```python
from build123d import *

# Parameters (mm, degrees)
F0_W      = 63.5
F0_H      = 6.35
F1_DEPTH  = 38.1
F2_W      = 25.4
F2_H      = 38.1
F3_DEPTH  = 12.7
F5_DEPTH  = 25.4
F6_R      = 6.35
F7_DEPTH  = 25.4
F9_DEPTH  = 25.4
F11_DEPTH = 12.7
F12_R     = 3.4395833333
F13_DEPTH = 25.4
F14_DEPTH = 25.4


with BuildPart() as f1:
    # F0 (on Front) → F1 (new body)
    with BuildSketch(Plane.XZ):
        with Locations((-14.0939018427, 3.175)):
            Rectangle(F0_W, F0_H)
    extrude(amount=F1_DEPTH)

    # F2 (on face) → F3 (join)
    with BuildSketch(Plane(origin=(0, 0, 0), x_dir=(-1, 0, 0), z_dir=(0, 1, 0))):
        with Locations((33.1439018427, 25.4)):
            Rectangle(F2_W, F2_H)
    extrude(amount=-F3_DEPTH)

    # F4 (on face) → F5 (cut)
    with BuildSketch(Plane.XZ.offset(12.7)):
        with BuildLine():
            ThreePointArc((-45.8439018427, 25.4), (-33.1439018427, 38.1), (-20.4439018427, 25.4))
            Line((-20.4439018427, 25.4), (-20.4439018427, 44.45))
            Line((-20.4439018427, 44.45), (-45.8439018427, 44.45))
            Line((-45.8439018427, 44.45), (-45.8439018427, 25.4))
        make_face()
    extrude(amount=-F5_DEPTH, mode=Mode.SUBTRACT)

    # F6 (on face) → F7 (cut)
    with BuildSketch(Plane.XZ.offset(12.7)):
        with Locations((-33.1439018427, 25.4)):
            Circle(F6_R)
    extrude(amount=-F7_DEPTH, mode=Mode.SUBTRACT)

    # F8 (on face) → F9 (cut)
    with BuildSketch(Plane.XZ.offset(12.7)):
        with BuildLine():
            add(Edge.make_bspline(
                [(-20.4439018427, 25.4), (-21.2112794526, 20.9739528082), (-22.6711814471, 15.8700383759), (-20.4439018427, 12.7)],
                knots=[0, 0, 0, 0, 0.4860571438, 0.4860571438, 0.4860571438, 0.4860571438], degree=3))
            Line((-20.4439018427, 12.7), (-20.4439018427, 25.4))
        make_face()
    extrude(amount=-F9_DEPTH, mode=Mode.SUBTRACT)

    # F10 (on face) → F11 (join)
    with BuildSketch(Plane.XZ.offset(12.7)):
        with BuildLine():
            add(Edge.make_bspline(
                [(-20.4439018427, 12.7), (-18.2158628234, 9.3571333053), (-12.2381824129, 8.0261796099), (-7.7439018427, 6.35)],
                knots=[0.4860571438, 0.4860571438, 0.4860571438, 0.4860571438, 1, 1, 1, 1], degree=3))
            Line((-20.4439018427, 12.7), (-20.4439018427, 6.35))
            Line((-20.4439018427, 6.35), (-7.7439018427, 6.35))
        make_face()
    extrude(amount=-F11_DEPTH)

    # F12 (on face) → F13 (cut)
    with BuildSketch(Plane.XY.offset(6.35)):
        with Locations((8.1310981573, -9.2604166667)):
            Circle(F12_R)
    extrude(amount=-F13_DEPTH, mode=Mode.SUBTRACT)

    # F14 (cut): a face of the model
    f14_faces = [f1.faces().sort_by_distance(p)[0] for p in [
        (-11.2918846227, -22.4788355031, 6.35),
    ]]
    extrude(f14_faces, amount=-F14_DEPTH, mode=Mode.SUBTRACT)


solid = f1.part
```
Source: CAD feature listing. Evaluate the final solid. Frame: model axes, mm. Coordinates: 2 decimals unless noted, no trailing zeros. Loops run counter-clockwise (first coordinate to the right, second up) from the corner with the lowest first, then second, coordinate; pieces in that order, holes last. Notation, with made-up numbers: M 76,-22.5 L 91,-22.5 A17 ccw 91,-11.5 Z; hole C 32.25,88.25 d10. An arc over 180 degrees is marked long. Use CSV: the item, a comma, the result in double quotes.
(1) Draft query along Z for faces 1 (the face through (-31, -12.7, 15)), 2 (the face through (-38.183, -6.439, 21.536)), 3 (the face through (-27, -6, 0)). Return one class per face: pulls with the +Z half, pulls with the -Z half, needs draft (parallel to the pull), parting line crosses it, or undercut.
Answers follow:
face 1,"needs draft"
face 2,"undercut"
face 3,"pulls with the -Z half"
(2) Cut plane C-C on x = -40. Return loops of the section in (y, z), and give its area (3 significant figures).
Answers follow:
outline,"M -12.7,0 L 0,0 L 0,36.09 L -12.7,36.09 Z"
area,"458 mm²"
(3) Contact query for flat-ended pins moving along their axis: pin 1 (3 mm diameter, centred on x = -40, y = -8, fed in from +Z); pin 2 (1 mm diameter, centred on y = -4, z = 12, fed in from +X); pin 3 (4 mm diameter, centred on x = -14.5, y = -10.5, fed in from +Z). Output: stop coordinate, or through.
Answers follow:
pin 1,"z = 36.92"
pin 2,"x = -19.4"
pin 3,"z = 9.6"
(4) Cut plane B-B on z = 31. Return loops of the section in (x, y), and give its area (3 significant figures).
Answers follow:
outline,"M -44.54,-12.7 L -36.14,-12.7 L -36.14,0 L -44.54,0 Z; M -30.15,-12.7 L -21.75,-12.7 L -21.75,0 L -30.15,0 Z"
area,"213 mm²"
(5) Cut plane A-A on x = -35. Return loops of the section in (y, z), and give its area (3 significant figures).
Answers follow:
outline,"M -12.7,0 L 0,0 L 0,19.33 L -12.7,19.33 Z; M -12.7,31.47 L 0,31.47 L 0,37.96 L -12.7,37.96 Z"
area,"328 mm²"
(6) Line query: line 1 (X direction, y = -2.25, z = 31); line 2 (X direction, y = -2.25, z = 26.5); line 3 (Z direction, x = -39, y = -9). Output: solid intervals per line, ascending. Write a range as [from, to].
Answers follow:
line 1,"[-44.54, -36.14], [-30.15, -21.75]"
line 2,"[-45.8, -39.4], [-26.89, -20.49]"
line 3,"[0, 22.94], [27.86, 36.67]"
